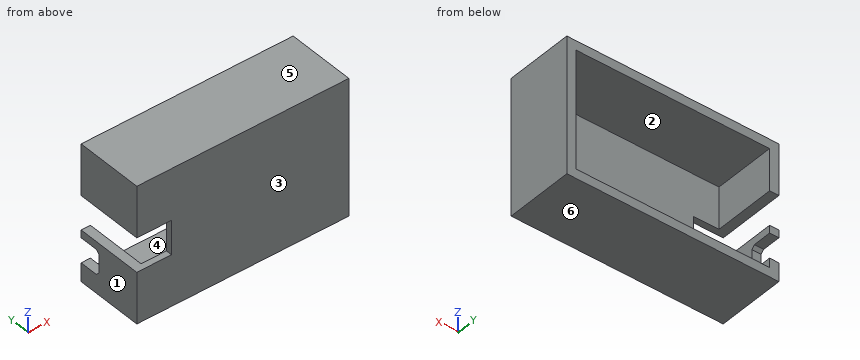
```python
from build123d import *

# Parameters (mm, degrees)
BOSS_EXTRUDE1_DEPTH = 20
SKETCH2_W           = 68.5
SKETCH2_H           = 44
BOSS_EXTRUDE2_DEPTH = 2
SKETCH3_W           = 11
SKETCH3_H           = 2
CUT_EXTRUDE1_DEPTH  = 11.2
SKETCH4_W           = 8
SKETCH4_H           = 7
CUT_EXTRUDE2_DEPTH  = 10
CHAMFER2_SIZE       = 1


with BuildPart() as part:
    # Sketch1 → Boss-Extrude1 (new body)
    with BuildSketch(Plane(origin=(0, 0, 0), x_dir=(1, 0, 0), z_dir=(0, 1, 0))):
        Polygon((-33.284090909, -14.318181818), (-33.284090909, -27.818181818), (29.215909091, -27.818181818), (29.215909091, 10.181818182), (-33.284090909, 10.181818182), (-33.284090909, -3.318181818), (-36.284090909, -3.318181818), (-36.284090909, 13.181818182), (32.215909091, 13.181818182), (32.215909091, -30.818181818), (-36.284090909, -30.818181818), (-36.284090909, -14.318181818), align=None)
    extrude(amount=BOSS_EXTRUDE1_DEPTH)

    # Sketch2 → Boss-Extrude2 (add)
    with BuildSketch(Plane.XZ):
        with Locations((-2.034090909, 8.818181818)):
            Rectangle(SKETCH2_W, SKETCH2_H)
    extrude(amount=BOSS_EXTRUDE2_DEPTH)

    # Sketch3 → Cut-Extrude1 (cut)
    with BuildSketch(Plane.ZY.offset(36.284090909)):
        with Locations((8.818181818, -1)):
            Rectangle(SKETCH3_W, SKETCH3_H)
    extrude(amount=-CUT_EXTRUDE1_DEPTH, mode=Mode.SUBTRACT)

    # Sketch4 → Cut-Extrude2 (cut)
    with BuildSketch(Plane(origin=(-33.284090909, 0, 0), x_dir=(0, 0, -1), z_dir=(1, 0, 0))):
        with Locations((3.181818182, 16.5)):
            Rectangle(SKETCH4_W, SKETCH4_H)
    extrude(amount=-CUT_EXTRUDE2_DEPTH, mode=Mode.SUBTRACT)

    # Chamfer2
    chamfer2_edges = [part.edges().sort_by_distance(p)[0] for p in [
        (-34.784090909, 13, -7.181818182),
        (-34.784090909, 13, 0.818181818),
    ]]
    chamfer(chamfer2_edges, length=CHAMFER2_SIZE)


solid = part.part
```
Design review of the part built by this model. Coordinates are the model's own, in mm. Face numbers are marked on the shaded views. A direction names the side the tool comes from. Give positions to 0.01 mm unless a question says otherwise; leave off trailing zeros. Write each loop counter-clockwise with the first axis right and the second up, starting at its lowest first coordinate (ties: lowest second). Pieces come first, ordered by that corner, then holes. Notation, with made-up numbers: (0, -21.5) -> (8, -21.5) arc R30 ccw to (8, 2.5) -> close; hole circle Ø7 at (21.5, 10). An arc over 180 degrees is marked (long way). Answer in a Markdown table with one row per item.
(1) Consider section D-D (y = 0.75). State the section outline as (x, z) points, then the cut area to 3 significant figures.
Results:
| item | result |
|---|---|
| outline | (-36.28, -13.18) -> (32.22, -13.18) -> (32.22, 30.82) -> (-36.28, 30.82) -> (-36.28, 14.32) -> (-33.28, 14.32) -> (-33.28, 27.82) -> (29.22, 27.82) -> (29.22, -10.18) -> (-33.28, -10.18) -> (-33.28, 3.32) -> (-36.28, 3.32) -> close |
| area | 606 mm2 |
(2) For the marked faces 1 and 2, list the 3-axis set-ups (+Z, -Z, +X, -X, +Y, -Y) from which the entire face can be reached by the end or side of a thin tool; tool diameter is ignored.
Results:
| item | result |
|---|---|
| face 1 | +Z, -Z, -X, +Y, -Y |
| face 2 | +Y |
(3) Consider section C-C (x = -4.5). State the section outline as (y, z) points, then the cut area to 3 significant figures.
Results:
| item | result |
|---|---|
| outline | (-2, -13.18) -> (20, -13.18) -> (20, -10.18) -> (0, -10.18) -> (0, 27.82) -> (20, 27.82) -> (20, 30.82) -> (-2, 30.82) -> close |
| area | 208 mm2 |
(4) To check wall thickness, follow probe 1 along Z at (x, y) = (-3, 10); probe 2 along X at (y, z) = (3, -8); probe 3 along Y at (x, z) = (-32, -4.5). State the ranges of each line that lie inside material, in increasing order.
Results:
| item | result |
|---|---|
| probe 1 | -13.18 to -10.18, 27.82 to 30.82 |
| probe 2 | -36.28 to -33.28, 29.22 to 32.22 |
| probe 3 | -2 to 0 |
(5) Clearance check with flat-ended pins moving along their axes: pin 1 (11.5 mm diameter, centred on x = -6, z = 15, fed in from +Y); pin 2 (0.9 mm diameter, centred on x = -35, z = -2.5, fed in from +Y); pin 3 (0.6 mm diameter, centred on y = -0.5, z = 6, fed in from -X). State where each tip first meets the part, or that it passes through.
Results:
| item | result |
|---|---|
| pin 1 | y = 0 |
| pin 2 | y = 13 |
| pin 3 | x = -25.08 |
(6) Consider section A-A (y = 18.5). State the section outline as (x, z) points.
Results:
| item | result |
|---|---|
| outline | (-36.28, -13.18) -> (32.22, -13.18) -> (32.22, 30.82) -> (-36.28, 30.82) -> (-36.28, 14.32) -> (-33.28, 14.32) -> (-33.28, 27.82) -> (29.22, 27.82) -> (29.22, -10.18) -> (-33.28, -10.18) -> (-33.28, -7.18) -> (-36.28, -7.18) -> close; (-36.28, 0.82) -> (-33.28, 0.82) -> (-33.28, 3.32) -> (-36.28, 3.32) -> close |
(7) Consider section B-B (z = 16.5). State the section outline as (x, y) points.
Results:
| item | result |
|---|---|
| outline | (-36.28, -2) -> (32.22, -2) -> (32.22, 20) -> (29.22, 20) -> (29.22, 0) -> (-33.28, 0) -> (-33.28, 20) -> (-36.28, 20) -> close |
(8) Mouldability with a two-part tool opening along Z and no side actions: class the marked faces 3, 4, 5 and 6 as +Z half, -Z half, draft (parallel to the pull), parting line (faces both ways), or undercut.
Results:
| item | result |
|---|---|
| face 3 | draft |
| face 4 | undercut |
| face 5 | +Z half |
| face 6 | -Z half |
